from build123d import *

# Parameters (mm, degrees)
SKETCH1_W                = 10
SKETCH1_H                = 6
BOSS_EXTRUDE1_DEPTH      = 15
BOSS_EXTRUDE1_2_DEPTH    = 15
FILLET1_R                = 5
FILLET2_R                = 5
BOSS_EXTRUDE2_DEPTH      = 3
BOSS_EXTRUDE2_DEPTH_BACK = 1
SKETCH2_W                = 10
SKETCH2_H                = 25
SKETCH3_R                = 1.6
CUT_EXTRUDE1_DEPTH       = 31.822070015
CUT_EXTRUDE2_REACH       = 34.388
SKETCH4_R                = 1.6
CHAMFER1_SIZE            = 1.5


with BuildPart() as part:
    # Sketch1 → Boss-Extrude1 (new body)
    with BuildSketch(Plane.XY):
        with Locations((5, 3)):
            Rectangle(SKETCH1_W, SKETCH1_H)
    extrude(amount=BOSS_EXTRUDE1_DEPTH)

    # Fillet2
    fillet2_edges = [part.edges().sort_by_distance(p)[0] for p in [
        (10, 3, 15),
        (0, 3, 15),
    ]]
    fillet(fillet2_edges, radius=FILLET2_R - 0.0001)  # a hair under: the kernel refuses the full size



with BuildPart() as body_2:
    # Sketch1 → Boss-Extrude1 2 (new body)
    with BuildSketch(Plane.XY):
        with Locations((5, 22)):
            Rectangle(SKETCH1_W, SKETCH1_H)
    extrude(amount=BOSS_EXTRUDE1_2_DEPTH)

    # Fillet1
    fillet1_edges = [body_2.edges().sort_by_distance(p)[0] for p in [
        (10, 22, 15),
        (0, 22, 15),
    ]]
    fillet(fillet1_edges, radius=FILLET1_R - 0.0001)  # a hair under: the kernel refuses the full size


with BuildPart() as part_1:
    add(part.part)

    add(body_2.part)  # Boss-Extrude2 merges body 2
    # Sketch2 → Boss-Extrude2 (add, two sides: drawn at the far end of the back side and taken through both)
    with BuildSketch(Plane(origin=(0, 0, 0), x_dir=(-1, 0, 0), z_dir=(0, 0, -1)).offset(-BOSS_EXTRUDE2_DEPTH_BACK)):
        with Locations((-5, 12.5)):
            Rectangle(SKETCH2_W, SKETCH2_H)
    extrude(amount=BOSS_EXTRUDE2_DEPTH + BOSS_EXTRUDE2_DEPTH_BACK)

    # Sketch3 → Cut-Extrude1 (cut, through all)
    with BuildSketch(Plane(origin=(0, 25, 0), x_dir=(1, 0, 0), z_dir=(0, 1, 0))):
        with Locations(Location((5, -10, 0), (0, 0, 270))):
            Circle(SKETCH3_R)
    extrude(amount=-CUT_EXTRUDE1_DEPTH, mode=Mode.SUBTRACT)

    # Sketch4 → Cut-Extrude2 (cut, up to next)
    with BuildSketch(Plane(origin=(0, 0, -3), x_dir=(-1, 0, 0), z_dir=(0, 0, -1)), mode=Mode.PRIVATE) as cut_extrude2_sk1:
        with Locations((-5, 12.5)):
            Circle(SKETCH4_R)
    cut_extrude2_tool1 = extrude(cut_extrude2_sk1.sketch, amount=-CUT_EXTRUDE2_REACH, mode=Mode.PRIVATE) & part_1.part
    add(cut_extrude2_tool1.solids().sort_by_distance((5, 12.5, -3))[0], mode=Mode.SUBTRACT)

    # Chamfer1
    chamfer1_edges = [part_1.edges().sort_by_distance(p)[0] for p in [
        (5, 6, 1),
        (5, 19, 1),
    ]]
    chamfer(chamfer1_edges, length=CHAMFER1_SIZE)


solid = part_1.part
Build history of the part. All positions in model axes, mm. A direction names the side the tool comes from. Round coordinates to 2 decimals unless told otherwise and drop trailing zeros. Write each loop counter-clockwise with the first axis right and the second up, starting at its lowest first coordinate (ties: lowest second). Pieces come first, ordered by that corner, then holes. Notation, with made-up numbers: M 63.5,37 L 106.5,37 A25 cw 106.5,74 Z; hole C 41.5,39 d6. An arc over 180 degrees is marked long. Answer as a JSON object with one key per item and string values. Group by question number.
(1) Which spindle directions (+Z, -Z, +X, -X, +Y, -Y) get a long thin tool onto all of the face, cutting with end or side? Do faces 4 (the cylindrical face through (9, 22, 13)), 5 (the flat face through (5.1, 18.3, 1.8)). Say none if no direction does.
(2) Drill centre lines: L1, parallel to Y at x = 4.25, z = 7.5; L2, parallel to X at y = 20.65, z = 10; L3, parallel to Z at x = 5, y = 15.5. Where is each one in solid material? Low to high.
(3) Mould opens along Y. For faces 1 (the flat face through (5, 25, 6)), 2 (the flat face through (0, 12.3, 0.7)), 3 (the flat face through (5.1, 6.7, 1.8)) say: pulls with the +Y half, pulls with the -Y half, needs draft (parallel to the pull), parting line crosses it, or undercut.
(4) Cut at A-A (z = 7.5). Give the cut face in (x, y).
(5) Cut at D-D (z = 10.5). Give the cut face in (x, y), and give its area (3 significant figures).
(6) Flat gauge pins, fed straight in: pin 1 (1 mm diameter, centred on y = 13.5, z = -1, fed in from -X); pin 2 (2.5 mm diameter, centred on x = 5, z = 10, fed in from -Y). Where does each tip first touch, or does it go through?
(7) Cut at B-B (y = 12.5). Give the cut face in (x, z), and give its area (3 significant figures).
Responses:
{
 "1": {"face 4": "+Z, +X, +Y, -Y", "face 5": "+Z, +X, -X"},
 "2": {"L1": "y = 0 to 6, 19 to 25", "L2": "x = 0 to 3.4, 6.6 to 10", "L3": "z = -3 to 1"},
 "3": {"face 1": "pulls with the +Y half", "face 2": "needs draft", "face 3": "undercut"},
 "4": {"outline": "M 0,0 L 10,0 L 10,6 L 0,6 Z; M 0,19 L 10,19 L 10,25 L 0,25 Z"},
 "5": {"outline": "M 0.03,0 L 3.48,0 L 3.48,6 L 0.03,6 Z; M 0.03,19 L 3.48,19 L 3.48,25 L 0.03,25 Z; M 6.52,0 L 9.97,0 L 9.97,6 L 6.52,6 Z; M 6.52,19 L 9.97,19 L 9.97,25 L 6.52,25 Z", "area": "82.9 mm2"},
 "6": {"pin 1": "stops at x = 0", "pin 2": "passes through"},
 "7": {"outline": "M 0,-3 L 3.4,-3 L 3.4,1 L 0,1 Z; M 6.6,-3 L 10,-3 L 10,1 L 6.6,1 Z", "area": "27.2 mm2"}
}
